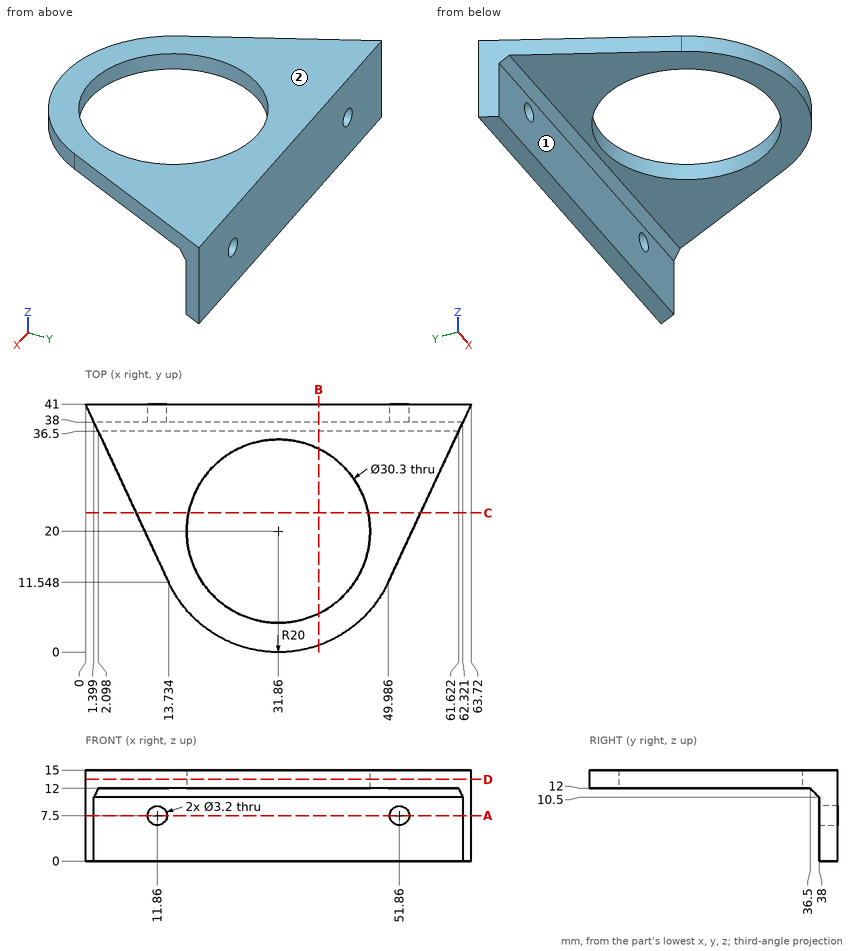
Could you check a few things on this drawing? It's one solid part, dimensions in mm from its lowest x, y, z. A direction names the side the tool comes from. Give positions to 0.01 mm unless a question says otherwise; leave off trailing zeros. Order: outer loops, then holes, each group sorted by start corner. A loop starts at its lowest first (then second) coordinate and runs counter-clockwise, first axis right, second up. Notation, with made-up numbers: (53, 10) -> (103, 10) arc R33 cw to (103, 41) -> close; hole circle Ø5 at (85.5, -23.75). An arc over 180 degrees is marked (long way). Answer in a Markdown table with one row per item. Add a question column.
Item 1: Imagine slicing it at B-B (x = 38.5). List the corners of the cut face in (y, z) for me (1 decimal).
Item 2: Imagine slicing it at C-C (y = 23). List the corners of the cut face in (x, z) for me, and give its area (3 significant figures).
Item 3: I'm going to push flat-ended pins straight in: P1, Ø5, axis at x = 10, y = 8.5, coming from the -Z side; P2, Ø18, axis at x = 21.5, y = 19, coming from the -Z side; P3, Ø8.5, axis at x = 32.5, z = 6, coming from the -Y side; P4, Ø8, axis at y = 32.5, z = 13.5, coming from the +X side. Where does each tip first touch, or does it pass through?
Item 4: Imagine slicing it at A-A (z = 7.5). List the corners of the cut face in (x, y) for me.
Item 5: For the marked faces 1 and 2, which set-ups out of +Z, -Z, +X, -X, +Y, -Y let a thin tool reach every point of the face, with its end or its side?
Item 6: Please list where these lines run through material, in increasing order: probe 1 along X at (y, z) = (39.45, 7.5); probe 2 along X at (y, z) = (39.8, 7.5); probe 3 along Y at (x, z) = (26, 6).
Item 7: Imagine slicing it at D-D (z = 13.5). List the corners of the cut face in (x, y) for me, and give its area (3 significant figures).
Result:
| question | item | result |
|---|---|---|
| 1 | outline | (1.1, 12) -> (6.4, 12) -> (6.4, 15) -> (1.1, 15) -> close; (33.6, 12) -> (36.5, 12) -> (38, 10.5) -> (38, 0) -> (41, 0) -> (41, 15) -> (33.6, 15) -> close |
| 2 | outline | (8.39, 12) -> (17.01, 12) -> (17.01, 15) -> (8.39, 15) -> close; (46.71, 12) -> (55.33, 12) -> (55.33, 15) -> (46.71, 15) -> close |
| 2 | area | 51.7 mm2 |
| 3 | P1 | through |
| 3 | P2 | z = 12 |
| 3 | P3 | y = 38 |
| 3 | P4 | x = 61.62 |
| 4 | outline | (0, 41) -> (1.4, 38) -> (10.26, 38) -> (10.26, 41) -> close; (13.46, 38) -> (50.26, 38) -> (50.26, 41) -> (13.46, 41) -> close; (53.46, 38) -> (62.32, 38) -> (63.72, 41) -> (53.46, 41) -> close |
| 5 | face 1 | -Z, +X, -X, -Y |
| 5 | face 2 | +Z, +X, -X, +Y, -Y |
| 6 | probe 1 | 0.72 to 10.26, 13.46 to 50.26, 53.46 to 63 |
| 6 | probe 2 | 0.56 to 10.26, 13.46 to 50.26, 53.46 to 63.16 |
| 6 | probe 3 | 38 to 41 |
| 7 | outline | (0, 41) -> (13.73, 11.55) arc R20 ccw to (49.99, 11.55) -> (63.72, 41) -> close; hole circle Ø30.3 at (31.86, 20) |
| 7 | area | 1,050 mm2 |
